For this review, take the finished solid that the model builds, in its own axes (mm). Face numbers are marked on the shaded views. A direction names the side the tool comes from. Round coordinates to 2 decimals unless told otherwise and drop trailing zeros. Write each loop counter-clockwise with the first axis right and the second up, starting at its lowest first coordinate (ties: lowest second). Pieces come first, ordered by that corner, then holes. Notation, with made-up numbers: (87.5, 48.5) -> (133.5, 48.5) arc R35 cw to (133.5, 86.5) -> close; hole circle Ø11 at (61, 70.25). An arc over 180 degrees is marked (long way). Answer as CSV lines item,"result". Start each with the question number.
Item 1: For pin 1 Ø2 at (y, z) = (8.5, 12) entering from +X, flat-tipped, find the tip position at first contact; note if it passes through.
Item 2: Wall thickness on probe 1 along Z at (x, y) = (1.4, 5.5); probe 2 along Z at (x, y) = (11, 1.3); probe 3 along Y at (x, z) = (10.5, 17): over which ranges is each line inside the solid? List them lowest first. Write a range as from..to.
Item 3: Take a section at A-A on z = 10. Give the boundary of the cut face in (x, y), then the cut area to 3 significant figures.
Item 4: Machinability: for the marked faces 1 and 2, which of the approach directions +Z, -Z, +X, -X, +Y, -Y give a long, thin tool a straight path to every point of the face, cutting with its end or side? Answer none if there is none.
Item 5: Take a section at B-B on x = 11. Give the boundary of the cut face in (y, z), then the cut area to 3 significant figures.
Item 6: Take a section at C-C on y = 5.5. Give the boundary of the cut face in (x, z).
Item 7: Take a section at D-D on y = 1. Give the boundary of the cut face in (x, z).
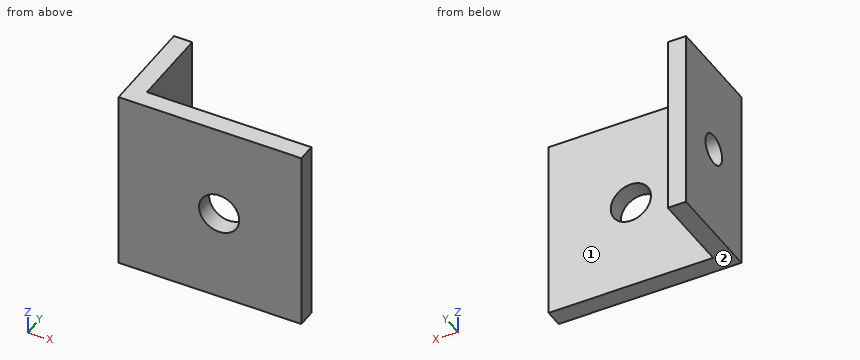
```python
from build123d import *

# Parameters (mm, degrees)
F1_DEPTH = 20
F3_D     = 4.4
F5_D     = 3.3


with BuildPart() as f1:
    # F0 (on Top) → F1 (new body)
    with BuildSketch(Plane.XY):
        Polygon((0, 11), (0, 0), (20, 0), (20, 2), (2, 2), (2, 11), align=None)
    extrude(amount=F1_DEPTH)

    # F3 (through all)
    with Locations(Plane(origin=(0, 2, 0), x_dir=(-1, 0, 0), z_dir=(0, 1, 0))):
        with Locations((-11, 10)):
            Hole(F3_D / 2)

    # F5 (through all)
    with Locations(Plane(origin=(0, 0, 0), x_dir=(0, -1, 0), z_dir=(-1, 0, 0))):
        with Locations((-5.5, 10)):
            Hole(F5_D / 2)


solid = f1.part
```
Output values:
1,pin 1,"stops at x = 2"
2,probe 1,"z = 0..8.35, 11.65..20"
2,probe 2,"z = 0..7.8, 12.2..20"
2,probe 3,"y = 0..2"
3,outline,"(0, 0) -> (8.8, 0) -> (8.8, 2) -> (2, 2) -> (2, 3.85) -> (0, 3.85) -> close; (0, 7.15) -> (2, 7.15) -> (2, 11) -> (0, 11) -> close; (13.2, 0) -> (20, 0) -> (20, 2) -> (13.2, 2) -> close"
3,area,"42.6 mm^2"
4,face 1,"+Z, -Z, +X, +Y"
4,face 2,"-Z, +X, -X, +Y, -Y"
5,outline,"(0, 0) -> (2, 0) -> (2, 7.8) -> (0, 7.8) -> close; (0, 12.2) -> (2, 12.2) -> (2, 20) -> (0, 20) -> close"
5,area,"31.2 mm^2"
6,outline,"(0, 0) -> (2, 0) -> (2, 8.35) -> (0, 8.35) -> close; (0, 11.65) -> (2, 11.65) -> (2, 20) -> (0, 20) -> close"
7,outline,"(0, 0) -> (20, 0) -> (20, 20) -> (0, 20) -> close; hole circle Ø4.4 at (11, 10)"
